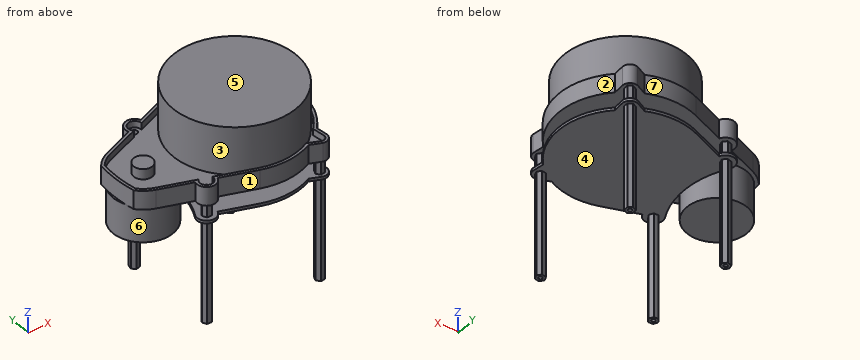
from build123d import *

# Parameters (mm, degrees)
ESQUISSE1_R             = 1.6
BOSS_EXTRU_1_DEPTH      = 10
ESQUISSE2_R             = 32.8
BOSS_EXTRU_2_DEPTH      = 22
ENL_V_MAT_EXTRU_1_DEPTH = 3.5
BOSS_EXTRU_3_REACH      = 79.261
ESQUISSE4_R             = 32.8
ESQUISSE5_R             = 16
BOSS_EXTRU_4_DEPTH      = 19
ESQUISSE6_R             = 1
BOSS_EXTRU_5_DEPTH      = 65
BOSS_EXTRU_6_DEPTH      = 1.5
ESQUISSE8_R             = 5
BOSS_EXTRU_7_DEPTH      = 5.5


with BuildPart() as part:
    # Esquisse1 → Boss.-Extru.1 (new body)
    with BuildSketch(Plane.XY):
        with BuildLine():
            ThreePointArc((-56.3, -16.861494596), (-60.528670487, -14.599558136), (-64.01, -11.301322931))
            ThreePointArc((-64.01, -11.301322931), (-65, 0), (-64.01, 11.301322931))
            ThreePointArc((-64.01, 11.301322931), (-60.528670487, 14.599558136), (-56.3, 16.861494596))
            Line((-56.3, 16.861494596), (-39.624688626, 23.091930519))
            ThreePointArc((-39.624688626, 23.091930519), (-36.690940127, 29.525679018), (-30.257191628, 26.591930519))
            Line((-30.257191628, 26.591930519), (-12.425, 33.254614341))
            ThreePointArc((-12.425, 33.254614341), (1.381675102, 35.473102119), (14.973963383, 32.187426436))
            Line((14.973963383, 32.187426436), (20.756023105, 34.801647207))
            ThreePointArc((20.756023105, 34.801647207), (24.347774736, 34.238511045), (26, 31))
            Line((26, 31), (25.359978077, 24.841930519))
            ThreePointArc((25.359978077, 24.841930519), (35.5, 0), (25.359978077, -24.841930519))
            Line((25.359978077, -24.841930519), (26, -31))
            ThreePointArc((26, -31), (24.347774736, -34.238511045), (20.756023105, -34.801647207))
            Line((20.756023105, -34.801647207), (14.973963383, -32.187426436))
            ThreePointArc((14.973963383, -32.187426436), (1.381675102, -35.473102119), (-12.425, -33.254614341))
            Line((-12.425, -33.254614341), (-30.257191628, -26.591930519))
            ThreePointArc((-30.257191628, -26.591930519), (-36.690940127, -29.525679018), (-39.624688626, -23.091930519))
            Line((-39.624688626, -23.091930519), (-56.3, -16.861494596))
        make_face()
        with Locations((-35, -25)):
            Circle(ESQUISSE1_R, mode=Mode.SUBTRACT)
        with Locations((22, 31)):
            Circle(ESQUISSE1_R, mode=Mode.SUBTRACT)
        with Locations((-35, 25)):
            Circle(ESQUISSE1_R, mode=Mode.SUBTRACT)
        with Locations((22, -31)):
            Circle(ESQUISSE1_R, mode=Mode.SUBTRACT)
    extrude(amount=BOSS_EXTRU_1_DEPTH)

    # Esquisse2 → Boss.-Extru.2 (add)
    with BuildSketch(Plane.XY.offset(10)):
        Circle(ESQUISSE2_R)
    extrude(amount=BOSS_EXTRU_2_DEPTH)

    # Esquisse3 → Enl_v. mat.-Extru.1 (cut)
    with BuildSketch(Plane.XY.offset(10)):
        with BuildLine():
            Line((-55.775, -15.456370046), (-37.378202776, -22.330008789))
            ThreePointArc((-37.378202776, -22.330008789), (-36.165940127, -28.120554469), (-31.453677478, -24.543603151))
            Line((-31.453677478, -24.543603151), (-11.9, -31.849489792))
            ThreePointArc((-11.9, -31.849489792), (1.664031028, -33.959255009), (14.956816294, -30.533484019))
            Line((14.956816294, -30.533484019), (21.291141631, -33.397398551))
            ThreePointArc((21.291141631, -33.397398551), (23.468656713, -33.023128137), (24.499056843, -31.06866508))
            Line((24.499056843, -31.06866508), (23.79417774, -24.286562245))
            ThreePointArc((23.79417774, -24.286562245), (34, 0), (23.79417774, 24.286562245))
            Line((23.79417774, 24.286562245), (24.499056843, 31.06866508))
            ThreePointArc((24.499056843, 31.06866508), (23.468656713, 33.023128137), (21.291141631, 33.397398551))
            Line((21.291141631, 33.397398551), (14.956816294, 30.533484019))
            ThreePointArc((14.956816294, 30.533484019), (1.664031028, 33.959255009), (-11.9, 31.849489792))
            Line((-11.9, 31.849489792), (-31.453677478, 24.543603151))
            ThreePointArc((-31.453677478, 24.543603151), (-36.165940127, 28.120554469), (-37.378202776, 22.330008789))
            Line((-37.378202776, 22.330008789), (-55.775, 15.456370046))
            ThreePointArc((-55.775, 15.456370046), (-59.496201473, 13.493411636), (-62.6, 10.653168543))
            ThreePointArc((-62.6, 10.653168543), (-63.5, 0), (-62.6, -10.653168543))
            ThreePointArc((-62.6, -10.653168543), (-59.496201473, -13.493411636), (-55.775, -15.456370046))
        make_face()
    extrude(amount=-ENL_V_MAT_EXTRU_1_DEPTH, mode=Mode.SUBTRACT)


with BuildPart() as enl_v_mat_extru_1_piece_1:
    # of the separate pieces the step leaves, piece 1, a body of its own (enl_v_mat_extru_1_pieces)
    add(part.part.solids().sort_by_distance((32.8, 0, 10))[0])


with BuildPart() as enl_v_mat_extru_1_piece_2:
    # of the separate pieces the step leaves, piece 2, a body of its own (enl_v_mat_extru_1_pieces)
    add(part.part.solids().sort_by_distance((-64.01, 11.301322931, 0))[0])

    # Esquisse4 → Boss.-Extru.3 (add, up to next)
    with BuildSketch(Plane(origin=(0, 0, 10), x_dir=(-1, 0, 0), z_dir=(0, 0, -1)), mode=Mode.PRIVATE) as boss_extru_3_sk1:
        with Locations(Location((0, 0, 0), (0, 0, 180))):
            Circle(ESQUISSE4_R)
    boss_extru_3_tool1 = extrude(boss_extru_3_sk1.sketch, amount=BOSS_EXTRU_3_REACH, mode=Mode.PRIVATE) - enl_v_mat_extru_1_piece_2.part

    add(enl_v_mat_extru_1_piece_1.part)  # Boss.-Extru.3 merges Enl_v. mat.-Extru.1 piece 1
    add(boss_extru_3_tool1.solids().sort_by_distance((0, 0, 10))[0])

    # Esquisse5 → Boss.-Extru.4 (add)
    with BuildSketch(Plane(origin=(0, 0, 0), x_dir=(-1, 0, 0), z_dir=(0, 0, -1))):
        with Locations(Location((50, 0, 0), (0, 0, 336.653490915))):
            Circle(ESQUISSE5_R)
    extrude(amount=BOSS_EXTRU_4_DEPTH)

    # Esquisse6 → Boss.-Extru.5 (add)
    # profile 1 of 4: a face of its own
    with BuildSketch(Plane(origin=(0, 0, 0), x_dir=(-1, 0, 0), z_dir=(0, 0, -1))):
        Polygon((-20.489225606, -29.008126327), (-22.969626005, -28.695694159), (-24.480400399, -30.687567832), (-23.510774394, -32.991873673), (-21.030373995, -33.304305841), (-19.519599601, -31.312432168), align=None)
        with Locations((-22, -31)):
            Circle(ESQUISSE6_R, mode=Mode.SUBTRACT)
    # profile 2 of 4: a face of its own
    with BuildSketch(Plane(origin=(0, 0, 0), x_dir=(-1, 0, 0), z_dir=(0, 0, -1))):
        Polygon((36.086835018, -22.748602735), (33.593650283, -22.933074633), (32.506815266, -25.184471898), (33.913164982, -27.251397265), (36.406349717, -27.066925367), (37.493184734, -24.815528102), align=None)
        with Locations((35, -25)):
            Circle(ESQUISSE6_R, mode=Mode.SUBTRACT)
    # profile 3 of 4: a face of its own
    with BuildSketch(Plane(origin=(0, 0, 0), x_dir=(-1, 0, 0), z_dir=(0, 0, -1))):
        Polygon((36.720274889, 26.814016072), (34.289153443, 27.396809791), (32.568878555, 25.582793719), (33.279725111, 23.185983928), (35.710846557, 22.603190209), (37.431121445, 24.417206281), align=None)
        with Locations((35, 25)):
            Circle(ESQUISSE6_R, mode=Mode.SUBTRACT)
    # profile 4 of 4: a face of its own
    with BuildSketch(Plane(origin=(0, 0, 0), x_dir=(-1, 0, 0), z_dir=(0, 0, -1))):
        Polygon((-19.952160425, 32.43399898), (-22.217959758, 33.490480585), (-24.265799333, 32.056481605), (-24.047839575, 29.56600102), (-21.782040242, 28.509519415), (-19.734200667, 29.943518395), align=None)
        with Locations((-22, 31)):
            Circle(ESQUISSE6_R, mode=Mode.SUBTRACT)
    extrude(amount=BOSS_EXTRU_5_DEPTH)

    # Esquisse7 → Boss.-Extru.6 (add)
    with BuildSketch(Plane(origin=(0, 0, -8), x_dir=(-1, 0, 0), z_dir=(0, 0, -1))):
        with BuildLine():
            Line((30.257191628, 26.591930519), (12.425, 33.254614341))
            ThreePointArc((12.425, 33.254614341), (-1.381675102, 35.473102119), (-14.973963383, 32.187426436))
            Line((-14.973963383, 32.187426436), (-20.756023105, 34.801647207))
            ThreePointArc((-20.756023105, 34.801647207), (-24.347774736, 34.238511045), (-26, 31))
            Line((-26, 31), (-25.359978077, 24.841930519))
            ThreePointArc((-25.359978077, 24.841930519), (-35.5, 0), (-25.359978077, -24.841930519))
            Line((-25.359978077, -24.841930519), (-26, -31))
            ThreePointArc((-26, -31), (-24.347774736, -34.238511045), (-20.756023105, -34.801647207))
            Line((-20.756023105, -34.801647207), (-14.973963383, -32.187426436))
            ThreePointArc((-14.973963383, -32.187426436), (-1.381675102, -35.473102119), (12.425, -33.254614341))
            Line((12.425, -33.254614341), (30.257191628, -26.591930519))
            ThreePointArc((30.257191628, -26.591930519), (36.690940127, -29.525679018), (39.624688626, -23.091930519))
            ThreePointArc((39.624688626, -23.091930519), (33.487603548, 0), (39.624688626, 23.091930519))
            ThreePointArc((39.624688626, 23.091930519), (36.690940127, 29.525679018), (30.257191628, 26.591930519))
        make_face()
    extrude(amount=BOSS_EXTRU_6_DEPTH)

    # Esquisse8 → Boss.-Extru.7 (add)
    with BuildSketch(Plane.XY.offset(6.5)):
        with Locations((-50, 0)):
            Circle(ESQUISSE8_R)
    extrude(amount=BOSS_EXTRU_7_DEPTH)


solid = enl_v_mat_extru_1_piece_2.part
Build history of the part. All positions in model axes, mm. Face numbers are marked on the shaded views. A direction names the side the tool comes from. Round coordinates to 2 decimals unless told otherwise and drop trailing zeros. Order: outer loops, then holes, each group sorted by start corner. A loop starts at its lowest first (then second) coordinate and runs counter-clockwise, first axis right, second up. Notation, with made-up numbers: M -12,11.5 L 44,11.5 A20 ccw 44,34.5 Z; hole C 77,64.5 d5. An arc over 180 degrees is marked long. Use CSV: the item, a comma, the result in double quotes. Start each with the question number.
(1) Tool access for the marked faces 1, 2, 3 and 4: list every direction of +Z, -Z, +X, -X, +Y, -Y with a clear straight run to the whole face (end or side of a thin tool).
(2) Cut at C-C on y = 13. List the corners of the cut face in (x, z).
(3) Cut at D-D on x = -59. List the corners of the cut face in (y, z), then the cut area to 3 significant figures.
(4) Mould opens along Y. For the marked faces 5, 6 and 7 say: +Y half, -Y half, draft (parallel to the pull), parting line (faces both ways), or undercut.
(5) Drill centre lines: probe 1 along Z at (x, y) = (7, -7.5); probe 2 along Y at (x, z) = (-35.5, -59.5); probe 3 along Y at (x, z) = (-30, 8). Where is each one in solid material? Low to high.
(6) Flat gauge pins, fed straight in: P1, Ø1.6, axis at x = 22.5, y = 31, coming from the +Z side; P2, Ø3, axis at x = -52, y = -1, coming from the +Z side; P3, Ø0.6, axis at x = 22.5, y = -31, coming from the +Z side; P4, Ø6, axis at y = -12, z = -23, coming from the +X side. Where does each tip first touch, or does it go through?
(7) Cut at A-A on x = 0. List the corners of the cut face in (y, z).
(8) Cut at B-B on z = -24.5. List the corners of the cut face in (x, y), then the cut area to 3 significant figures.
Findings:
1,face 1,"+Z, -Z, -Y"
1,face 2,"+Z, -Z, +X"
1,face 3,"+Z"
1,face 4,"-Z"
2,outline,"M -62.45,0 L -59.33,0 L -59.33,-19 L -40.67,-19 L -40.67,0 L 33.03,0 L 33.03,10 L 31.42,10 L 31.42,6.5 L 30.11,6.5 L 30.11,32 L -30.11,32 L -30.11,6.5 L -60.16,6.5 L -60.16,10 L -62.45,10 Z; M -35.34,-9.5 L 33.03,-9.5 L 33.03,-8 L -35.34,-8 Z"
3,outline,"M -15.59,0 L -13.23,0 L -13.23,-19 L 13.23,-19 L 13.23,0 L 15.59,0 L 15.59,10 L 13.83,10 L 13.83,6.5 L -13.83,6.5 L -13.83,10 L -15.59,10 Z"
3,area,"718 mm^2"
4,face 5,"draft"
4,face 6,"undercut"
4,face 7,"+Y half"
5,probe 1,"z = -9.5 to -8, 0 to 32"
5,probe 2,"y = -27.13 to -25.87, -24.13 to -22.79, 22.65 to 24.13, 25.87 to 27.11"
5,probe 3,"y = -26.69 to -25.09, -13.26 to 13.26, 25.09 to 26.69"
6,P1,"stops at z = 0"
6,P2,"stops at z = 12"
6,P3,"stops at z = -8"
6,P4,"passes through"
7,outline,"M -35.5,-9.5 L 35.5,-9.5 L 35.5,-8 L -35.5,-8 Z; M -35.5,0 L 35.5,0 L 35.5,10 L 34,10 L 34,6.5 L 32.8,6.5 L 32.8,32 L -32.8,32 L -32.8,6.5 L -34,6.5 L -34,10 L -35.5,10 Z"
8,outline,"M -37.49,-24.82 L -36.41,-27.07 L -33.91,-27.25 L -32.51,-25.18 L -33.59,-22.93 L -36.09,-22.75 Z; M -37.43,24.42 L -35.71,22.6 L -33.28,23.19 L -32.57,25.58 L -34.29,27.4 L -36.72,26.81 Z; M 19.52,-31.31 L 21.03,-33.3 L 23.51,-32.99 L 24.48,-30.69 L 22.97,-28.7 L 20.49,-29.01 Z; M 19.73,29.94 L 21.78,28.51 L 24.05,29.57 L 24.27,32.06 L 22.22,33.49 L 19.95,32.43 Z; hole C -35,-25 d2; hole C -35,25 d2; hole C 22,-31 d2; hole C 22,31 d2"
8,area,"52.4 mm^2"
